For this review, take the finished solid that the model builds, in its own axes (mm). Coordinates: 2 decimals unless noted, no trailing zeros. Loops run counter-clockwise (first coordinate to the right, second up) from the corner with the lowest first, then second, coordinate; pieces in that order, holes last. Notation, with made-up numbers: (16.5, 21.25) -> (50.5, 21.25) arc R17 cw to (50.5, 36.25) -> close; hole circle Ø8 at (36, 36). An arc over 180 degrees is marked (long way). One line per item, written item: value.
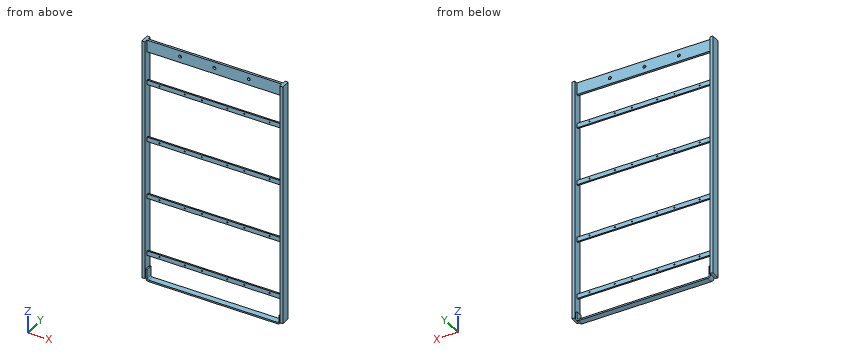
from build123d import *

# Parameters (mm, degrees)
F0_W     = 572.516
F0_H     = 50.8
F1_DEPTH = 4.5593
F2_DEPTH = 19.05
F3_R     = 6.35
F4_DEPTH = 25.4
F6_W     = 572.516
F6_H     = 19.05
F6_R     = 2.54
F7_DEPTH = 3.175
F8_DEPTH = 12.7


with BuildPart() as f1:
    # F0 (on Front) → F1 (new body, symmetric)
    with BuildSketch(Plane.XZ):
        with Locations((0, 489.5977)):
            Rectangle(F0_W, F0_H)
    extrude(amount=F1_DEPTH, both=True)

    # F0 (on Front) → F2 (join, symmetric)
    with BuildSketch(Plane.XZ):
        Polygon((-286.258, 464.1977), (-286.258, 514.9977), (-298.958, 514.9977), (-298.958, -514.9977), (-286.258, -514.9977), align=None)
        Polygon((298.958, 514.9977), (286.258, 514.9977), (286.258, 464.1977), (286.258, -514.9977), (298.958, -514.9977), align=None)
    extrude(amount=F2_DEPTH, both=True)

    # F3 (on face) → F4 (cut)
    with BuildSketch(Plane.XZ.offset(4.5593)):
        with Locations((146.05, 489.5977)):
            Circle(F3_R)
        with Locations((-146.05, 489.5977)):
            Circle(F3_R)
        with Locations((0, 489.5977)):
            Circle(F3_R)
    extrude(amount=-F4_DEPTH, mode=Mode.SUBTRACT)

    # F6 (on Front) → F7 (join, symmetric)
    with BuildSketch(Plane.XZ):
        with Locations((0, -412.7627)):
            Rectangle(F6_W, F6_H)
        with Locations((-233.7562, -412.7627)):
            Circle(F6_R, mode=Mode.SUBTRACT)
        with Locations((-126.2634, -412.7627)):
            Circle(F6_R, mode=Mode.SUBTRACT)
        with Locations((-53.7464, -412.7627)):
            Circle(F6_R, mode=Mode.SUBTRACT)
        with Locations((53.7464, -412.7627)):
            Circle(F6_R, mode=Mode.SUBTRACT)
        with Locations((126.2634, -412.7627)):
            Circle(F6_R, mode=Mode.SUBTRACT)
        with Locations((233.7562, -412.7627)):
            Circle(F6_R, mode=Mode.SUBTRACT)
        with Locations((0, -165.1127)):
            Rectangle(F6_W, F6_H)
        with Locations((-233.7562, -165.1127)):
            Circle(F6_R, mode=Mode.SUBTRACT)
        with Locations((-126.2634, -165.1127)):
            Circle(F6_R, mode=Mode.SUBTRACT)
        with Locations((-53.7464, -165.1127)):
            Circle(F6_R, mode=Mode.SUBTRACT)
        with Locations((53.7464, -165.1127)):
            Circle(F6_R, mode=Mode.SUBTRACT)
        with Locations((126.2634, -165.1127)):
            Circle(F6_R, mode=Mode.SUBTRACT)
        with Locations((233.7562, -165.1127)):
            Circle(F6_R, mode=Mode.SUBTRACT)
        with Locations((0, 82.5373)):
            Rectangle(F6_W, F6_H)
        with Locations((-233.7562, 82.5373)):
            Circle(F6_R, mode=Mode.SUBTRACT)
        with Locations((-126.2634, 82.5373)):
            Circle(F6_R, mode=Mode.SUBTRACT)
        with Locations((-53.7464, 82.5373)):
            Circle(F6_R, mode=Mode.SUBTRACT)
        with Locations((53.7464, 82.5373)):
            Circle(F6_R, mode=Mode.SUBTRACT)
        with Locations((126.2634, 82.5373)):
            Circle(F6_R, mode=Mode.SUBTRACT)
        with Locations((233.7562, 82.5373)):
            Circle(F6_R, mode=Mode.SUBTRACT)
        with Locations((0, 330.1873)):
            Rectangle(F6_W, F6_H)
        with Locations((-233.7562, 330.1873)):
            Circle(F6_R, mode=Mode.SUBTRACT)
        with Locations((-126.2634, 330.1873)):
            Circle(F6_R, mode=Mode.SUBTRACT)
        with Locations((-53.7464, 330.1873)):
            Circle(F6_R, mode=Mode.SUBTRACT)
        with Locations((53.7464, 330.1873)):
            Circle(F6_R, mode=Mode.SUBTRACT)
        with Locations((126.2634, 330.1873)):
            Circle(F6_R, mode=Mode.SUBTRACT)
        with Locations((233.7562, 330.1873)):
            Circle(F6_R, mode=Mode.SUBTRACT)
    extrude(amount=F7_DEPTH, both=True)

    # F5 (on Front) → F8 (join, symmetric)
    with BuildSketch(Plane.XZ):
        with BuildLine():
            Line((-279.9461, -476.8977), (-286.2961, -476.8977))
            Line((-286.2961, -476.8977), (-286.2961, -514.9977))
            ThreePointArc((-286.2961, -514.9977), (-282.576356, -523.977956), (-273.5961, -527.6977))
            Line((-273.5961, -527.6977), (273.5961, -527.6977))
            ThreePointArc((273.5961, -527.6977), (282.576356, -523.977956), (286.2961, -514.9977))
            Line((286.2961, -514.9977), (286.2961, -487.987315))
            Line((286.2961, -487.987315), (279.9461, -487.987315))
            Line((279.9461, -487.987315), (279.9461, -514.9977))
            ThreePointArc((279.9461, -514.9977), (278.086228, -519.487828), (273.5961, -521.3477))
            Line((273.5961, -521.3477), (-273.5961, -521.3477))
            ThreePointArc((-273.5961, -521.3477), (-278.086228, -519.487828), (-279.9461, -514.9977))
            Line((-279.9461, -514.9977), (-279.9461, -476.8977))
        make_face()
    extrude(amount=F8_DEPTH, both=True)


solid = f1.part
1. Take a section at B-B, the plane z = -318.5. Give the boundary of the cut face in (x, y).
Return value:
outline: (-298.96, -19.05) -> (-286.26, -19.05) -> (-286.26, 19.05) -> (-298.96, 19.05) -> close; (286.26, -19.05) -> (298.96, -19.05) -> (298.96, 19.05) -> (286.26, 19.05) -> close
2. Insertion check: pin 1 Ø3 at (x, z) = (-126.26, -165.11) entering from +Y; pin 2 Ø6.5 at (x, z) = (53.75, 330.19) entering from -Y (3 decimals); pin 3 Ø1.5 at (x, y) = (158.5, -12) entering from +Z; pin 4 Ø6 at (x, z) = (-126.26, -412.76) entering from +Y (3 decimals). Each pin has a flat end and moves straight along its axis. Give the tip position at first contact, or say it passes through.
Return value:
pin 1: passes through
pin 2: stops at y = -3.175
pin 3: stops at z = -521.35
pin 4: stops at y = 3.175
3. To check wall thickness, follow probe 1 along Z at (x, y) = (24.5, 1.5); probe 2 along X at (y, z) = (10.5, -91); probe 3 along Z at (x, y) = (10, 4). State the ranges of each line that lie inside material, in increasing order. Write a range as from..to.
Return value:
probe 1: z = -527.7..-521.35, -422.29..-403.24, -174.64..-155.59, 73.01..92.06, 320.66..339.71, 464.2..515
probe 2: x = -298.96..-286.26, 286.26..298.96
probe 3: z = -527.7..-521.35, 464.2..515
4. Take a section at A-A, the plane x = 250. Give the boundary of the cut face in (y, z) (3 decimals).
Return value:
outline: (-12.7, -527.698) -> (12.7, -527.698) -> (12.7, -521.348) -> (-12.7, -521.348) -> close; (-4.559, 464.198) -> (4.559, 464.198) -> (4.559, 514.998) -> (-4.559, 514.998) -> close; (-3.175, -422.288) -> (3.175, -422.288) -> (3.175, -403.238) -> (-3.175, -403.238) -> close; (-3.175, -174.638) -> (3.175, -174.638) -> (3.175, -155.588) -> (-3.175, -155.588) -> close; (-3.175, 73.012) -> (3.175, 73.012) -> (3.175, 92.062) -> (-3.175, 92.062) -> close; (-3.175, 320.662) -> (3.175, 320.662) -> (3.175, 339.712) -> (-3.175, 339.712) -> close
